Autodesk Inventor part; units mm, degrees
ref_plane "YZ Plane" through (0, 0, 0) normal (1, 0, 0) x (0, 1, 0)
ref_plane "XZ Plane" through (0, 0, 0) normal (0, 1, 0) x (-1, 0, 0)
ref_plane "XY Plane" through (0, 0, 0) normal (0, 0, 1) x (1, 0, 0)
sketch "Sketch1" plane through (0, 0, 0) normal (0, 1, 0) x (-1, 0, 0)
  line L0 (31.4392, 172.5) -> (-79.5, 172.5)
  line L1 (-34.5, -172.5) -> (31.4392, -172.5)
  line L2 (102.5, -107.5) -> (102.5, 107.5)
  line L3 (102.5, 172.5) -> (-102.5, -172.5) construction
  line L4 (-102.5, 172.5) -> (102.5, -172.5) construction
  line L5 (-132.5, 55) -> (-207.5, 55)
  line L6 (-217.5, 45) -> (-217.5, -45)
  line L7 (-217.5, -55) -> (-132.5, -55)
  line L8 (41.929, 166.3277) -> (60.071, 133.6723)
  line L9 (70.5608, 127.5) -> (82.5, 127.5)
  line L10 (102.5, 0) -> (-217.5, 0)
  line L11 (41.929, -166.3277) -> (60.071, -133.6723)
  line L12 (70.5608, -127.5) -> (82.5, -127.5)
  circle A0 centre (-208.1, 0) radius 3
  arc A1 (102.5, 107.5) -> (82.5, 127.5) centre (82.5, 107.5) ccw
  arc A2 (82.5, -127.5) -> (102.5, -107.5) centre (82.5, -107.5) ccw
  line L13 (-102.5, 149.5) -> (-102.5, 85)
  line L14 (-102.5, -85) -> (-102.5, -149.5)
  arc A3 (-132.5, 55) -> (-102.5, 85) centre (-132.5, 85) ccw
  arc A4 (-102.5, -85) -> (-132.5, -55) centre (-132.5, -85) ccw
  arc A5 (-79.5, 172.5) -> (-102.5, 149.5) centre (-79.5, 149.5) ccw
  arc A6 (-102.5, -149.5) -> (-79.5, -172.5) centre (-79.5, -149.5) ccw
  circle A7 centre (-55.1, -158) radius 3
  circle A8 centre (-55.1, 158) radius 3
  circle A9 centre (52.5, 0) radius 40
  circle A10 centre (83.489, 30.989) radius 1.85
  line L15 (52.5, 0) -> (83.489, 30.989)
  circle A11 centre (21.511, 30.989) radius 1.85
  circle A12 centre (21.511, -30.989) radius 1.85
  circle A13 centre (83.489, -30.989) radius 1.85
  circle A14 centre (-32.5, 0) radius 40
  circle A15 centre (-1.511, 30.989) radius 1.85
  line L16 (-32.5, 0) -> (-1.511, 30.989)
  circle A16 centre (-63.489, 30.989) radius 1.85
  circle A17 centre (-63.489, -30.989) radius 1.85
  circle A18 centre (-1.511, -30.989) radius 1.85
  circle A19 centre (-117.5, 0) radius 40
  circle A20 centre (-86.511, 30.989) radius 1.85
  line L17 (-117.5, 0) -> (-86.511, 30.989)
  circle A21 centre (-148.489, 30.989) radius 1.85
  circle A22 centre (-148.489, -30.989) radius 1.85
  circle A23 centre (-86.511, -30.989) radius 1.85
  circle A24 centre (54.5, 80) radius 28.5
  line L18 (54.5, 80) -> (83, 80)
  line L19 (54.5, 80) -> (74.6525, 100.1525)
  circle A25 centre (77.3749, 102.8749) radius 1.85
  circle A26 centre (31.6251, 102.8749) radius 1.85
  circle A27 centre (31.6251, 57.1251) radius 1.85
  circle A28 centre (77.3749, 57.1251) radius 1.85
  circle A29 centre (-12.5, 80) radius 28.5
  line L20 (-12.5, 80) -> (16, 80)
  line L21 (-12.5, 80) -> (7.6525, 100.1525)
  circle A30 centre (10.3749, 102.8749) radius 1.85
  circle A31 centre (-35.3749, 102.8749) radius 1.85
  circle A32 centre (-35.3749, 57.1251) radius 1.85
  circle A33 centre (10.3749, 57.1251) radius 1.85
  circle A34 centre (54.5, -80) radius 28.5
  line L22 (54.5, -80) -> (83, -80)
  line L23 (54.5, -80) -> (74.6525, -59.8475)
  circle A35 centre (77.3749, -57.1251) radius 1.85
  circle A36 centre (31.6251, -57.1251) radius 1.85
  circle A37 centre (31.6251, -102.8749) radius 1.85
  circle A38 centre (77.3749, -102.8749) radius 1.85
  circle A39 centre (-12.5, -80) radius 28.5
  line L24 (-12.5, -80) -> (16, -80)
  line L25 (-12.5, -80) -> (7.6525, -59.8475)
  circle A40 centre (10.3749, -57.1251) radius 1.85
  circle A41 centre (-35.3749, -57.1251) radius 1.85
  circle A42 centre (-35.3749, -102.8749) radius 1.85
  circle A43 centre (10.3749, -102.8749) radius 1.85
  line L26 (-197, -25) -> (-163, -25)
  line L27 (-163, -25) -> (-163, 25)
  line L28 (-163, 25) -> (-197, 25)
  line L29 (-197, 25) -> (-197, -25)
  line L30 (-197, -25) -> (-163, 25) construction
  line L31 (-163, -25) -> (-197, 25) construction
  circle A44 centre (-17.5, 127.5) radius 6
  circle A45 centre (2.5, 127.5) radius 6
  circle A46 centre (22.5, 127.5) radius 6
  circle A47 centre (42.5, 127.5) radius 6
  line L32 (-79.5, -127.5) -> (-79.5, -100)
  line L33 (-124.5, -55) -> (-217.5, -55)
  line L34 (-79.5, -172.5) -> (31.4392, -172.5)
  arc A48 (-79.5, -100) -> (-124.5, -55) centre (-124.5, -100) ccw
  arc A49 (-79.5, -127.5) -> (-34.5, -172.5) centre (-34.5, -127.5) ccw
  line L35 (-34.5, 172.5) -> (31.4392, 172.5)
  line L36 (-79.5, 127.5) -> (-79.5, 100)
  line L37 (-124.5, 55) -> (-217.5, 55)
  arc A50 (-124.5, 55) -> (-79.5, 100) centre (-124.5, 100) ccw
  arc A51 (-34.5, 172.5) -> (-79.5, 127.5) centre (-34.5, 127.5) ccw
  arc A52 (31.4392, -172.5) -> (41.929, -166.3277) centre (31.4392, -160.5) ccw
  arc A53 (41.929, 166.3277) -> (31.4392, 172.5) centre (31.4392, 160.5) ccw
  arc A54 (70.5608, -127.5) -> (60.071, -133.6723) centre (70.5608, -139.5) ccw
  arc A55 (60.071, 133.6723) -> (70.5608, 127.5) centre (70.5608, 139.5) ccw
  line L38 (-47.5, -115.6878) -> (-47.5, -100)
  line L39 (-92.5, -55) -> (-207.5, -55)
  line L40 (-47.5, -172.5) -> (31.4392, -172.5)
  line L41 (-48.0352, -119.2314) -> (-61.6974, -163.4329)
  arc A56 (-47.5, -100) -> (-92.5, -55) centre (-92.5, -100) ccw
  arc A57 (-48.0352, -119.2314) -> (-47.5, -115.6878) centre (-59.5, -115.6878) ccw
  line L42 (-55.0096, -172.5) -> (31.4392, -172.5)
  arc A58 (-61.6974, -163.4329) -> (-55.0096, -172.5) centre (-55.0096, -165.5) ccw
  line L43 (-47.5, 115.6878) -> (-47.5, 100)
  line L44 (-92.5, 55) -> (-217.5, 55)
  line L45 (-48.0352, 119.2314) -> (-61.6974, 163.4329)
  arc A59 (-92.5, 55) -> (-47.5, 100) centre (-92.5, 100) ccw
  arc A60 (-47.5, 115.6878) -> (-48.0352, 119.2314) centre (-59.5, 115.6878) ccw
  line L46 (-55.0096, 172.5) -> (31.4392, 172.5)
  arc A61 (-55.0096, 172.5) -> (-61.6974, 163.4329) centre (-55.0096, 165.5) ccw
  circle A62 centre (102.5, 46) radius 4
  circle A63 centre (102.5, -49) radius 3
  circle A64 centre (-37.5, 127.5) radius 3.5
  arc A65 (-217.5, -45) -> (-207.5, -55) centre (-207.5, -45) ccw
  arc A66 (-207.5, 55) -> (-217.5, 45) centre (-207.5, 45) ccw
  circle A67 centre (42.5, -127.5) radius 3.5
  circle A68 centre (22.5, -127.5) radius 3.5
  circle A69 centre (2.5, -127.5) radius 3.5
  circle A70 centre (-17.5, -127.5) radius 3.5
  line L47 (-124.5, 55) -> (-132.5, 55)
  line L48 (-34.5, 172.5) -> (-79.5, 172.5)
  arc A71 (-61.6767, 163.3668) -> (-61.6974, 163.4329) centre (-55.0096, 165.5) ccw
  arc A72 (-61.6767, 163.3668) -> (-79.5, 127.5) centre (-34.5, 127.5) ccw
  line L49 (-79.5, 127.5) -> (-79.5, 100)
  line L50 (-61.6974, 163.4329) -> (-47.6345, 117.4797)
  line L51 (-47.5, 100) -> (-47.6345, 117.4797)
  line L52 (-92.5, 55) -> (-124.5, 55)
  line L53 (-92.5, 55) -> (-124.5, 55)
  line L54 (-92.5, 55) -> (-124.5, 55)
  line L55 (-55.0096, 172.5) -> (-79.5, 172.5)
  line L56 (-34.5, 172.5) -> (-55.0096, 172.5)
  arc A73 (-34.5, 172.5) -> (-61.6771, 163.3665) centre (-34.5, 127.5) ccw
  arc A74 (-55.0096, 172.5) -> (-61.6766, 163.3666) centre (-55.0096, 165.5) ccw
  point P0 (0, 0)
  point P1 (-102.5, 55)
  point P2 (63.5, 127.5)
  point P3 (38.5, 172.5)
  point P4 (102.5, 127.5)
  point P5 (63.5, -127.5)
  point P6 (38.5, -172.5)
  point P7 (102.5, -127.5)
  point P8 (-102.5, -55)
  point P9 (-12.5, 101)
  point P10 (69.5, -67.7951)
  point P11 (-13.8374, -72.5218)
  point P12 (-180, 0)
  point P13 (-47.5, -117.5)
  point P14 (-64.5, -172.5)
  dimension "d0" = 345
  dimension "d1" = 205
  dimension "d2" = 110
  dimension "d4" = 55
  dimension "d5" = 141
  dimension "d6" = 45
  dimension "d7" = 25
  dimension "d8" = 172.5
  dimension "d9" = 102.5
  dimension "d10" = 320
  dimension "d11" = 9.4
  dimension "d12" = 6
  dimension "d13" = 20
  dimension "d14" = 20
  dimension "d15" = 115
  dimension "d16" = 115
  dimension "d17" = 30
  dimension "d18" = 23
  dimension "d19" = 153
  dimension "d20" = 158
  dimension "d21" = 6
  dimension "d22" = 80
  dimension "d23" = 3.7
  dimension "d24" = 43.825
  dimension "d25" = 45
  dimension "d28" = 360
  dimension "d30" = 50
  dimension "d33" = 80
  dimension "d34" = 3.7
  dimension "d35" = 43.825
  dimension "d36" = 360
  dimension "d41" = 80
  dimension "d42" = 3.7
  dimension "d43" = 43.825
  dimension "d44" = 360
  dimension "d45" = 135
  dimension "d46" = 220
  dimension "d50" = 45
  dimension "d51" = 85
  dimension "d52" = 85
  dimension "d53" = 57
  dimension "d54" = 45
  dimension "d55" = 3.7
  dimension "d56" = 3.85
  dimension "d59" = 360
  dimension "d61" = 80
  dimension "d62" = 48
  dimension "d71" = 57
  dimension "d72" = 45
  dimension "d73" = 3.7
  dimension "d74" = 3.85
  dimension "d75" = 360
  dimension "d86" = 57
  dimension "d87" = 45
  dimension "d88" = 3.7
  dimension "d89" = 3.85
  dimension "d90" = 360
  dimension "d103" = 57
  dimension "d104" = 45
  dimension "d105" = 3.7
  dimension "d106" = 3.85
  dimension "d107" = 360
  dimension "d108" = 115
  dimension "d109" = 115
extrude "Extrusion1" add sketch "Sketch1" along normal blind 3 contours A53 L8 A55 L9 A1 L2 A62 L10 A9 A14 A19 L27 L28 L29 A0 L6 A66 L5 L37 L44 A59 L43 A60 L45 A71 A8 A51 L0 | A51 A71 A61 L0 | A61 L45 A51 L36 A50 L37 A3 L13 A5 L0 | A71 A8 A51 | A51 L45 A71 | L50 L51 A59 L44 A50 L36 A51 | L45 A60 L50 | A60 L43 L51 | L2 A62 | L2 A63 A2 L12 A54 L11 A52 L1 A49 L41 A57 L38 A56 L39 L33 L7 A65 L6 L10 A0 L29 L26 L27 A19 A14 A9 | L2 A63 | A9 L10 | L10 L15 A9 | A0 L10 | L10 A0 | L10 A9 L15 | A14 L10 | L10 L16 A14 | L29 L28 L27 L10 | L10 L27 L26 L29 | L10 A14 L16 | A19 L10 | L10 L17 A19 | A19 L17 L10 | A58 L41 A49 L34 picked at (102.1809, 47.2946) picked at (101.5073, -49.1205)
extrude "Extrusion2" cut sketch "Sketch1" along normal blind 3 contours A9 L10 | L10 L15 A9 | L10 A9 L15 | A14 L10 | L10 L16 A14 | L29 L28 L27 L10 | L10 L27 L26 L29 | L10 A14 L16 | A19 L10 | L10 L17 A19 | A19 L17 L10
extrude "Extrusion3" cut sketch "Sketch1" along normal blind 3 contours A62 L2 | L2 A62 | A63 L2 | L2 A63
extrude "Extrusion4" cut sketch "Sketch1" along normal blind 3 contours A0 L10 | L10 A0
extrude "Extrusion12" cut sketch "Sketch1" along normal blind 10 contours A51 A71 A61 L0 | A61 L45 A51 L36 A50 L37 A3 L13 A5 L0 | A51 L45 A71 | L50 L51 A59 L44 A50 L36 A51
extrude "Extrusion13" add sketch "Sketch1" along normal blind 3 contours A51 A71 A61 L0 | A51 L45 A71
properties part number "instrument_panel"
Geometry check sheet. Reference: the model listing, model coordinates, mm. A direction names the side the tool comes from. Round coordinates to 2 decimals unless told otherwise and drop trailing zeros. Order: outer loops, then holes, each group sorted by start corner. A loop starts at its lowest first (then second) coordinate and runs counter-clockwise, first axis right, second up. Notation, with made-up numbers: (36, -28) - (66, -28) arc R13 ccw to (66, -14) - close; hole circle Ø6 at (29, 89.25). An arc over 180 degrees is marked (long way). Use a Markdown table: item, result. Add a question column.
(1) Depth check by flat-ended pin: pin 1 (5.5 mm diameter, centred on x = -2.5, z = -127.5, fed in from -Y) (1 decimal); pin 2 (0.9 mm diameter, centred on x = -76.5, y = 1.5, fed in from +Z); pin 3 (1 mm diameter, centred on x = 144, y = 2, fed in from -Z); pin 4 (5 mm diameter, centred on x = -31.63, z = -102.87, fed in from -Y). Enter the tip coordinate at first touch or a pass-through.
(2) Material ranges on line 1 along X through (y, z) = (1.95, -80); line 2 along Z through (x, y) = (169, 2.25); line 3 along Z through (x, y) = (90, 2.7), recorded low to high. Write a range as [from, to].
(3) Sectioned sample at A-A, the plane x = 141.5. Enter the section's corners in (y, z).
(4) Sectioned sample at B-B, the plane z = 90. Enter the section's corners in (x, y), and give its area (3 significant figures).
(5) Sectioned sample at D-D, the plane y = 1.65. Count the separate pieces of the cut face and the enclosed holes in it, and give its area (3 significant figures).
(6) Tool access check on faces 5 (the flat face through (54.754, 1.479, 140.744)), 6 (the cylindrical face through (18.68, 1.48, 107.82)). Record the directions out of +Z, -Z, +X, -X, +Y, -Y that give a thin tool (end or side, any length) a straight path to the whole face; none if there is none.
(7) Release check for a two-part mould opening along X. For faces 1 (the flat face through (-11, 0, 2)), 2 (the cylindrical face through (61.032, 1.479, -67.832)), 3 (the cylindrical face through (-37.74, 1.48, 131.15)), 4 (the cylindrical face through (2.26, 1.48, 131.15)) record: pulls with the +X half, pulls with the -X half, needs draft (parallel to the pull), parting line crosses it, or undercut.
(8) Sectioned sample at C-C, the plane x = -54.5. Enter the section's corners in (y, z).
Answers below:
| question | item | result |
|---|---|---|
| 1 | pin 1 | through |
| 1 | pin 2 | z = 127.5 |
| 1 | pin 3 | z = -55 |
| 1 | pin 4 | y = 0 |
| 2 | line 1 | [-102.5, -83], [-26, -16], [41, 52.19] |
| 2 | line 2 | [-55, -25], [25, 55] |
| 2 | line 3 | [-55.07, -29.05], [29.05, 55.07] |
| 3 | outline | (0, -55) - (3, -55) - (3, -32) - (0, -32) - close; (0, 32) - (3, 32) - (3, 55) - (0, 55) - close |
| 4 | outline | (-102.5, 0) - (-81.19, 0) - (-81.19, 3) - (-102.5, 3) - close; (-27.81, 0) - (-14.19, 0) - (-14.19, 3) - (-27.81, 3) - close; (39.19, 0) - (48.63, 0) - (48.63, 3) - (39.19, 3) - close |
| 4 | area | 133 mm² |
| 5 | separate pieces | 1 |
| 5 | enclosed holes | 48 |
| 5 | area | 39,300 mm² |
| 6 | face 5 | +X, +Y, -Y |
| 6 | face 6 | +Y, -Y |
| 7 | face 1 | needs draft |
| 7 | face 2 | pulls with the +X half |
| 7 | face 3 | undercut |
| 7 | face 4 | undercut |
| 8 | outline | (0, -143.7) - (3, -143.7) - (3, -108.5) - (0, -108.5) - close; (0, -51.5) - (3, -51.5) - (3, -39.95) - (0, -39.95) - close; (0, 39.95) - (3, 39.95) - (3, 51.5) - (0, 51.5) - close; (0, 108.5) - (3, 108.5) - (3, 143.7) - (0, 143.7) - close |
